Design review of the part built by this model. Coordinates are the model's own, in mm. A direction names the side the tool comes from. Round coordinates to 2 decimals unless told otherwise and drop trailing zeros. Order: outer loops, then holes, each group sorted by start corner. A loop starts at its lowest first (then second) coordinate and runs counter-clockwise, first axis right, second up. Notation, with made-up numbers: (-13.75, -22.5) - (38.25, -22.5) arc R17 cw to (38.25, -11.5) - close; hole circle Ø4 at (77, 60). An arc over 180 degrees is marked (long way). Use CSV: the item, a comma, the result in double quotes.
from build123d import *

# Parameters (mm, degrees)
SKETCH2_R           = 6
BOSS_EXTRUDE1_DEPTH = 5.6
SKETCH3_R           = 6
SKETCH3_R_2         = 5.3
CUT_EXTRUDE1_DEPTH  = 4.4
FILLET1_R           = 0.5
SKETCH4_W           = 5
SKETCH4_H           = 5
SKETCH4_W_2         = 4
SKETCH4_H_2         = 4
BOSS_EXTRUDE2_DEPTH = 2.5


with BuildPart() as part:
    # Sketch2 → Boss-Extrude1 (new body)
    with BuildSketch(Plane(origin=(0, 0, 0), x_dir=(1, 0, 0), z_dir=(0, 1, 0))):
        Circle(SKETCH2_R)
    extrude(amount=BOSS_EXTRUDE1_DEPTH)

    # Sketch3 → Cut-Extrude1 (cut)
    with BuildSketch(Plane(origin=(0, 5.6, 0), x_dir=(1, 0, 0), z_dir=(0, 1, 0))):
        Circle(SKETCH3_R)
        Circle(SKETCH3_R_2, mode=Mode.SUBTRACT)
    extrude(amount=-CUT_EXTRUDE1_DEPTH, mode=Mode.SUBTRACT)

    # Fillet1
    fillet1_edges = [part.edges().sort_by_distance(p)[0] for p in [
        (-5.3, 5.6, 0),
    ]]
    fillet(fillet1_edges, radius=FILLET1_R)

    # Sketch4 → Boss-Extrude2 (add)
    with BuildSketch(Plane.XZ):
        Rectangle(SKETCH4_W, SKETCH4_H)
        Rectangle(SKETCH4_W_2, SKETCH4_H_2, mode=Mode.SUBTRACT)
    extrude(amount=BOSS_EXTRUDE2_DEPTH)


solid = part.part
1) Insertion check: pin 1 Ø4 at (x, y) = (4, 3) entering from -Z; pin 2 Ø2 at (y, z) = (-1.5, -1) entering from +X; pin 3 Ø6 at (x, z) = (-4.5, 3.5) entering from +Y; pin 4 Ø1.2 at (x, y) = (1, -1.5) entering from -Z. Each pin has a flat end and moves straight along its axis. Give the tip position at first contact, or say it passes through.
Data:
pin 1,"stops at z = -5.12"
pin 2,"stops at x = 2.5"
pin 3,"stops at y = 5.6"
pin 4,"stops at z = -2.5"
2) We need section B-B (z = 0). Give the boundary of the cut face in (x, y), then the cut area to 3 significant figures.
Data:
outline,"(-6, 0) - (-2.5, 0) - (-2.5, -2.5) - (-2, -2.5) - (-2, 0) - (2, 0) - (2, -2.5) - (2.5, -2.5) - (2.5, 0) - (6, 0) - (6, 1.2) - (5.3, 1.2) - (5.3, 5.1) arc R0.5 ccw to (4.8, 5.6) - (-4.8, 5.6) arc R0.5 ccw to (-5.3, 5.1) - (-5.3, 1.2) - (-6, 1.2) - close"
area,"63.4 mm2"
3) The part is to be moulded in two halves that separate along Z. For faces 1 (the face through (0, -1, 2.5)), 2 (the face through (4.896, 3.177, 2.03)), 3 (the face through (3, 0, 0)), 4 (the face through (-2, -1, 0)), say which applies: +Z half, -Z half, draft (parallel to the pull), parting line (faces both ways), or undercut.
Data:
face 1,"+Z half"
face 2,"parting line"
face 3,"draft"
face 4,"undercut"
4) To check wall thickness, follow L1, parallel to Z at x = 0.5, y = -2; L2, parallel to Y at x = -2.25, z = -3.25; L3, parallel to Z at x = 2.25, y = 3. State the ranges of each line that lie inside material, in increasing order. Write a range as from..to.
Data:
L1,"z = -2.5..-2, 2..2.5"
L2,"y = 0..5.6"
L3,"z = -4.8..4.8"
5) For faces 5 (the face through (0, -1, -2.5)), 6 (the face through (4, 1.2, 4)), 7 (the face through (2.5, -1, 0)), 8 (the face through (0, -1, -2)), list the 3-axis set-ups (+Z, -Z, +X, -X, +Y, -Y) from which the entire face can be reached by the end or side of a thin tool; tool diameter is ignored.
Data:
face 5,"-Z, +X, -X, -Y"
face 6,"+Y"
face 7,"+Z, -Z, +X, -Y"
face 8,"-Y"
6) We need section A-A (x = 0). Give the boundary of the cut face in (y, z).
Data:
outline,"(-2.5, -2.5) - (0, -2.5) - (0, -6) - (1.2, -6) - (1.2, -5.3) - (5.1, -5.3) arc R0.5 ccw to (5.6, -4.8) - (5.6, 4.8) arc R0.5 ccw to (5.1, 5.3) - (1.2, 5.3) - (1.2, 6) - (0, 6) - (0, 2.5) - (-2.5, 2.5) - (-2.5, 2) - (0, 2) - (0, -2) - (-2.5, -2) - close"
7) We need section C-C (y = 3.5). Give the boundary of the cut face in (x, z).
Data:
outline,"circle Ø10.6 at (0, 0)"
